```python
from build123d import *


with BuildPart() as f1:
    # F0 (on Front) → F1 (revolve)
    with BuildSketch(Plane.XZ):
        with BuildLine():
            Line((0, 40.816609), (0, 0))
            Line((0, 0), (17.611366, 0))
            ThreePointArc((17.611366, 0), (17.993982, 0.325532), (17.733942, 0.755353))
            Line((17.733942, 0.755353), (8.418861, 3.86038))
            ThreePointArc((8.418861, 3.86038), (5.943789, 5.680245), (5, 8.603796))
            Line((5, 8.603796), (5, 39.806811))
            ThreePointArc((5, 39.806811), (5.208859, 40.696651), (5.791815, 41.40064))
            ThreePointArc((5.791815, 41.40064), (15.556327, 53.192449), (19.054722, 68.097269))
            Line((19.054722, 68.097269), (18.054722, 68.097269))
            ThreePointArc((18.054722, 68.097269), (14.660757, 53.637369), (5.187723, 42.197554))
            Line((5.187723, 42.197554), (0, 40.816609))
        make_face()
    revolve(axis=Axis((0, 0, 20.408305), (0, 0, 1)))


solid = f1.part
```
Geometry: final body of the model. Coordinates: model frame, mm. A direction names the side the tool comes from. Give positions to 0.01 mm unless a question says otherwise; leave off trailing zeros. Write each loop counter-clockwise with the first axis right and the second up, starting at its lowest first coordinate (ties: lowest second). Pieces come first, ordered by that corner, then holes.
1. Section query A-A, the plane z = 37.5. Return loops of the section in (x, y).
2. Draft query along X for faces 1 (the conical face through (0.24, 0.076, 40.884)), 2 (the conical face through (-1.9, -8.7, 3.7)), 3 (the flat face through (0, 0, 0)). Return one class per face: released by +X, released by -X, zero draft, split by the parting line, or undercut.
3. Section query B-B, the plane z = 5.5. Return loops of the section in (x, y), then the cut area to 3 significant figures.
4. Reachability of faces 4 (the cylindrical face through (-1.08, -4.88, 24.42)), 5 (the flat face through (7, -17, 68.097)) from +Z, -Z, +X, -X, +Y, -Y: full face, straight path, thin tool, end or side. Return the list, or none.
5. Pin query (flat end, axial travel): P1, Ø1.5, axis at x = 6, z = 45, coming from the -Y side; P2, Ø3, axis at x = 3.5, z = 28.5, coming from the +Y side; P3, Ø4, axis at x = -3, z = 24.5, coming from the -Y side; P4, Ø10, axis at x = 13.5, z = 27, coming from the +Y side. Return the tip coordinate at first contact, or that it passes through.
6. Line query: probe 1 along Z at (x, y) = (9.5, -5.5); probe 2 along X at (y, z) = (6.5, 60); probe 3 along Z at (x, y) = (0.5, -13.5). Output: solid intervals per line, ascending.
Computed:
1. outline: circle Ø10 at (0, 0)
2. face 1: undercut
2. face 2: split by the parting line
2. face 3: zero draft
3. outline: circle Ø12.16 at (0, 0)
3. area: 116 mm2
4. face 4: none
4. face 5: +Z, +X, -X, +Y, -Y
5. P1: stops at y = -8.77
5. P2: stops at y = 4.58
5. P3: stops at y = -4.9
5. P4: passes through
6. probe 1: z = 0 to 3.01, 46.28 to 47.85
6. probe 2: x = -16.85 to -15.74, 15.74 to 16.85
6. probe 3: z = 0 to 2.16, 49.64 to 51.52
